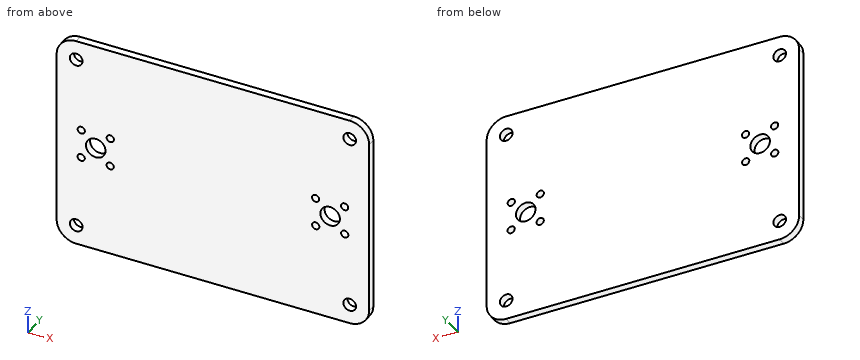
from build123d import *

# Parameters (mm, degrees)
SKETCH_1_R      = 5
SKETCH_1_R_2    = 1.85
SKETCH_1_R_3    = 3.25
EXTRUDE_1_DEPTH = 4


with BuildPart() as part:
    # Эскиз1 → Бобышка-Вытянуть1 (new body)
    with BuildSketch(Plane(origin=(0, 0, 0), x_dir=(1, 0, 0), z_dir=(0, 1, 0))):
        with BuildLine():
            Line((70, -55), (-70, -55))
            ThreePointArc((-70, -55), (-77.071067812, -52.071067812), (-80, -45))
            Line((-80, -45), (-80, 45))
            ThreePointArc((-80, 45), (-77.071067812, 52.071067812), (-70, 55))
            Line((-70, 55), (70, 55))
            ThreePointArc((70, 55), (77.071067812, 52.071067812), (80, 45))
            Line((80, 45), (80, -45))
            ThreePointArc((80, -45), (77.071067812, -52.071067812), (70, -55))
        make_face()
        with Locations((-60, 0)):
            Circle(SKETCH_1_R, mode=Mode.SUBTRACT)
        with Locations((-67.446640333, 7.402536575)):
            Circle(SKETCH_1_R_2, mode=Mode.SUBTRACT)
        with Locations((-52.597463425, 7.446640333)):
            Circle(SKETCH_1_R_2, mode=Mode.SUBTRACT)
        with Locations((-52.553359667, -7.402536575)):
            Circle(SKETCH_1_R_2, mode=Mode.SUBTRACT)
        with Locations((-67.402536575, -7.446640333)):
            Circle(SKETCH_1_R_2, mode=Mode.SUBTRACT)
        with Locations((52.597463425, 7.446640333)):
            Circle(SKETCH_1_R_2, mode=Mode.SUBTRACT)
        with Locations((52.553359667, -7.402536575)):
            Circle(SKETCH_1_R_2, mode=Mode.SUBTRACT)
        with Locations((67.402536575, -7.446640333)):
            Circle(SKETCH_1_R_2, mode=Mode.SUBTRACT)
        with Locations((60, 0)):
            Circle(SKETCH_1_R, mode=Mode.SUBTRACT)
        with Locations((67.446640333, 7.402536575)):
            Circle(SKETCH_1_R_2, mode=Mode.SUBTRACT)
        with Locations((-70, 45)):
            Circle(SKETCH_1_R_3, mode=Mode.SUBTRACT)
        with Locations((-70, -45)):
            Circle(SKETCH_1_R_3, mode=Mode.SUBTRACT)
        with Locations((70, -45)):
            Circle(SKETCH_1_R_3, mode=Mode.SUBTRACT)
        with Locations((70, 45)):
            Circle(SKETCH_1_R_3, mode=Mode.SUBTRACT)
    extrude(amount=EXTRUDE_1_DEPTH)


solid = part.part
Build history of the part. All positions in model axes, mm. Give positions to 0.01 mm unless a question says otherwise; leave off trailing zeros. Loops run counter-clockwise (first coordinate to the right, second up) from the corner with the lowest first, then second, coordinate; pieces in that order, holes last. Notation, with made-up numbers: (85, 67.25) - (99, 67.25) arc R19 cw to (99, 82.25) - close; hole circle Ø11 at (21.5, -15). An arc over 180 degrees is marked (long way). Write item = value, one per line. Start each with the question number.
1) Band-saw the part on B-B on x = -60. Give the cut face in (y, z).
2) Probe probe 1 along X at (y, z) = (3.1, 0); probe 2 along X at (y, z) = (1.05, 45); probe 3 along Z at (x, y) = (60, 1.2). List the from-to ranges inside material, lowest first. Write a range as from..to.
3) Drop a flat-ended pin along its axis: pin 1 Ø2 at (x, z) = (-52.55, 7.4) entering from +Y. Give the stop position or say it passes through.
4) Band-saw the part on A-A on z = 0. Give the cut face in (x, y), plus the area to 3 significant figures.
5) Band-saw the part on C-C on y = 0.95. Count the separate pieces of the cut face and the enclosed holes in it, plus the area to 3 significant figures.
Final values:
q1.outline = (0, -55) - (4, -55) - (4, -5) - (0, -5) - close; (0, 5) - (4, 5) - (4, 55) - (0, 55) - close
q2.probe_1 = -80..-65, -55..55, 65..80
q2.probe_2 = -80..-73.25, -66.75..66.75, 73.25..80
q2.probe_3 = -55..-5, 5..55
q3.pin_1 = through
q4.outline = (-80, 0) - (-65, 0) - (-65, 4) - (-80, 4) - close; (-55, 0) - (55, 0) - (55, 4) - (-55, 4) - close; (65, 0) - (80, 0) - (80, 4) - (65, 4) - close
q4.area = 560 mm²
q5.separate_pieces = 1
q5.enclosed_holes = 14
q5.area = 17,100 mm²
